CAD build for the part. Positions are in the model's coordinates, mm. A direction names the side the tool comes from. Round coordinates to 2 decimals unless told otherwise and drop trailing zeros. Loops run counter-clockwise (first coordinate to the right, second up) from the corner with the lowest first, then second, coordinate; pieces in that order, holes last. Notation, with made-up numbers: (-9, 83) - (39, 83) arc R20 ccw to (39, 97) - close; hole circle Ø11 at (9.25, 81). An arc over 180 degrees is marked (long way). Use one line per item in the form item = value.
Autodesk Inventor part; units mm, degrees
ref_plane "YZ Plane" through (0, 0, 0) normal (1, 0, 0) x (0, 1, 0)
ref_plane "XZ Plane" through (0, 0, 0) normal (0, 1, 0) x (-1, 0, 0)
ref_plane "XY Plane" through (0, 0, 0) normal (0, 0, 1) x (1, 0, 0)
sketch "Sketch1" plane through (0, 0, 0) normal (0, 1, 0) x (-1, 0, 0)
  arc A0 (0, -215.9) -> (152.6644, -152.6644) centre (0, 0) ccw
  arc A1 (0, -212.725) -> (150.4193, -150.4193) centre (0, 0) ccw
  line L0 (150.4193, -150.4193) -> (152.6644, -152.6644)
  line L1 (0, -212.725) -> (0, -215.9)
  dimension "d0" = 431.8
  dimension "d1" = 3.175
  dimension "d2" = 45
extrude "Extrusion1" add sketch "Sketch1" along normal blind 25.4
sketch "Sketch2" plane through (-150.4193, 0, -150.4193) normal (-0.7071, 0, 0.7071) x (0.7071, 0, 0.7071)
  line L0 (-3.175, 25.4) -> (0, 25.4)
  line L1 (0, 25.4) -> (0, 0)
  line L2 (0, 0) -> (-3.175, 0)
  line L3 (-3.175, 0) -> (-3.175, 25.4)
  point P0 (212.725, 0)
extrude "Extrusion2" add sketch "Sketch2" along normal blind 19.05
sketch "Sketch3" plane through (0, 0, -212.725) normal (1, 0, 0) x (0, 0, -1)
  line L0 (0, 0) -> (3.175, 0)
  line L1 (3.175, 0) -> (3.175, 25.4)
  line L2 (3.175, 25.4) -> (0, 25.4)
  line L3 (0, 25.4) -> (0, 0)
  point P0 (-212.725, 0)
extrude "Extrusion3" add sketch "Sketch3" along normal blind 19.05
properties part number "rail"
1) Drill centre lines: probe 1 along Z at (x, y) = (0.5, 12.25) (3 decimals); probe 2 along X at (y, z) = (14.5, -165.5); probe 3 along Z at (x, y) = (-54, 21.5). Where is each one in solid material? Low to high.
Report:
probe_1 = -215.9 to -212.725
probe_2 = -138.65 to -133.65
probe_3 = -209.04 to -205.76
2) Slice it at C-C (x = -129.5). Write the cut outline in (y, z), plus the area to 3 significant figures.
Report:
outline = (0, -172.75) - (25.4, -172.75) - (25.4, -168.77) - (0, -168.77) - close
area = 101 mm^2
3) Tool access for faces 1 (the flat face through (9, 13, -212.725)), 2 (the flat face through (-88, 25.4, -194)): list every direction of +Z, -Z, +X, -X, +Y, -Y with a clear straight run to the whole face (end or side of a thin tool).
Report:
face_1 = +Z, +X, +Y, -Y
face_2 = +Z, -Z, +X, -X, +Y
4) Flat gauge pins, fed straight in: pin 1 (12 mm diameter, centred on x = -105.5, z = -189.5, fed in from -Y); pin 2 (1 mm diameter, centred on x = -28, y = 12, fed in from +Z); pin 3 (10 mm diameter, centred on x = -70, y = 21, fed in from -Z); pin 4 (1 mm diameter, centred on y = 19, z = -177, fed in from -X). Where does each tip first touch, or does it go through?
Report:
pin_1 = 0
pin_2 = -210.81
pin_3 = -205.88
pin_4 = -124.34
5) Slice it at B-B (z = -202.5). Write the cut outline in (x, y).
Report:
outline = (-74.88, 0) - (-65.16, 0) - (-65.16, 25.4) - (-74.88, 25.4) - close
